```python
from build123d import *

# Parameters (mm, degrees)
F0_W     = 152.4
F0_H     = 228.6
F1_DEPTH = 1.5875
F2_W     = 76.2
F2_H     = 76.2
F3_DEPTH = 3.176
F4_W     = 3.175
F4_H     = 5.1537374914
F5_DEPTH = 10.16


with BuildPart() as f1:
    # F0 (on Front) → F1 (new body, symmetric)
    with BuildSketch(Plane.XZ):
        Rectangle(F0_W, F0_H)
    extrude(amount=F1_DEPTH, both=True)

    # F2 (on face) → F3 (cut, through all)
    with BuildSketch(Plane.XZ.offset(1.5875)):
        with Locations((38.1, 76.2)):
            Rectangle(F2_W, F2_H)
    extrude(amount=-F3_DEPTH, mode=Mode.SUBTRACT)

    # F4 (on face) → F5 (join)
    with BuildSketch(Plane.XZ.offset(1.5875)):
        with Locations((71.4375, 35.5231312543)):
            Rectangle(F4_W, F4_H)
    extrude(amount=F5_DEPTH)


solid = f1.part
```
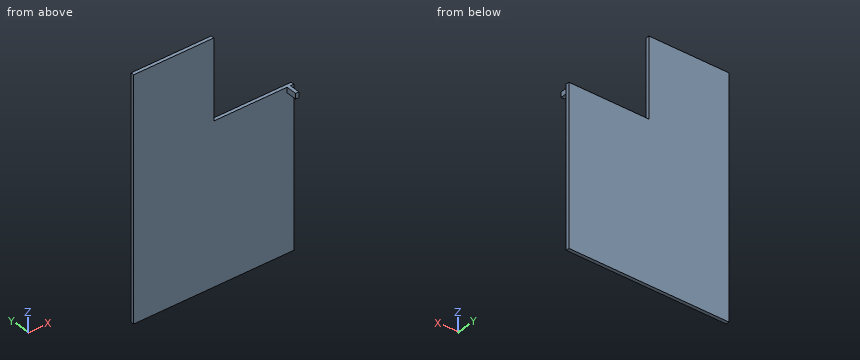
Part model, mm, in its own coordinate system. Round coordinates to 2 decimals unless told otherwise and drop trailing zeros. Order: outer loops, then holes, each group sorted by start corner. A loop starts at its lowest first (then second) coordinate and runs counter-clockwise, first axis right, second up. Notation, with made-up numbers: M 38.5,77 L 52.5,77 A25 ccw 52.5,97 Z; hole C 5.25,63 d1. An arc over 180 degrees is marked long. Put each result on its own line as item: value. Start each with the question number.
1. Slice it at B-B on z = 80.5. List the corners of the cut face in (x, y), then the cut area to 3 significant figures.
2. Drill centre lines: probe 1 along Y at (x, z) = (-20, 34); probe 2 along X at (y, z) = (-0.75, 80); probe 3 along X at (y, z) = (-5, 34) (3 decimals). Where is each one in solid material? Low to high. Write a range as [from, to].
3. Drop flat-ended pins along their axis: pin 1 (1.6 mm diameter, centred on x = 71, y = -8.5, fed in from -Z); pin 2 (6 mm diameter, centred on x = -60.5, z = 18, fed in from -Y); pin 3 (1.6 mm diameter, centred on y = 0, z = 71, fed in from +X). Give the stop position or say it passes through.
4. Slice it at A-A on x = 23. List the corners of the cut face in (y, z), then the cut area to 3 significant figures.
Findings:
1. outline: M -76.2,-1.59 L 0,-1.59 L 0,1.59 L -76.2,1.59 Z
1. area: 242 mm2
2. probe 1: [-1.59, 1.59]
2. probe 2: [-76.2, 0]
2. probe 3: [69.85, 73.025]
3. pin 1: z = 32.95
3. pin 2: y = -1.59
3. pin 3: x = 0
4. outline: M -1.59,-114.3 L 1.59,-114.3 L 1.59,38.1 L -1.59,38.1 Z
4. area: 484 mm2
